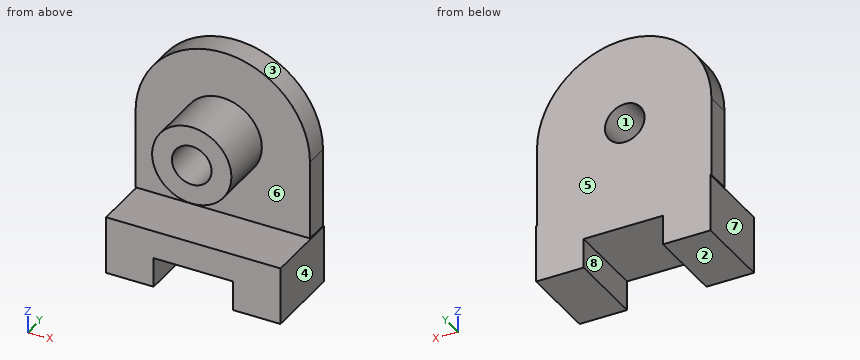
from build123d import *

# Parameters (mm, degrees)
F1_DEPTH = 12
F2_R     = 20
F3_DEPTH = 28
F5_DEPTH = 40
F6_R     = 10
F7_DEPTH = 70


with BuildPart() as f1:
    # F0 (on Front) → F1 (new body)
    with BuildSketch(Plane.XZ):
        with BuildLine():
            Line((44, 0), (44, 40))
            ThreePointArc((44, 40), (0, 84), (-44, 40))
            Line((-44, 40), (-44, 0))
            Line((-44, 0), (44, 0))
        make_face()
    extrude(amount=F1_DEPTH)

    # F2 (on face) → F3 (join)
    with BuildSketch(Plane.XZ.offset(12)):
        with Locations((-0.289364, 40.312858)):
            Circle(F2_R)
    extrude(amount=F3_DEPTH)

    # F4 (on Front) → F5 (join)
    with BuildSketch(Plane.XZ):
        Polygon((44.469752, -29.099998), (44.469752, 0), (-43.530248, 0), (-43.530248, -29.099998), (-19.530248, -29.099998), (-19.530248, -14.099998), (20.469752, -14.099998), (20.469752, -29.099998), align=None)
    extrude(amount=F5_DEPTH)

    # F6 (on face) → F7 (cut)
    with BuildSketch(Plane.XZ.offset(40)):
        with Locations((-0.289364, 40.312858)):
            Circle(F6_R)
    extrude(amount=-F7_DEPTH, mode=Mode.SUBTRACT)


solid = f1.part
The model under review builds one solid part; all positions refer to its coordinate system, in mm. Face numbers are marked on the shaded views. A direction names the side the tool comes from. Coordinates: 2 decimals unless noted, no trailing zeros. Loops run counter-clockwise (first coordinate to the right, second up) from the corner with the lowest first, then second, coordinate; pieces in that order, holes last. Notation, with made-up numbers: M -34.5,30.25 L -26.5,30.25 A24 cw -26.5,45.25 Z; hole C 6.25,-34.5 d1. An arc over 180 degrees is marked long. Put each result on its own line as item: value. Start each with the question number.
Q1. Add section D-D (x = -15). Write out the cut boundary in (y, z), and give its area (3 significant figures).
Q2. The part is to be moulded in two halves that separate along X. For the marked faces 1, 2, 3 and 4, say which applies: +X half, -X half, draft (parallel to the pull), parting line (faces both ways), or undercut.
Q3. Wall thickness on line 1 (Z direction, x = -1, y = -30); line 2 (Z direction, x = -35.5, y = -30.5); line 3 (X direction, y = -10, z = -12): over which ranges is each line inside the solid? List them lowest first.
Q4. Add section B-B (y = -20). Write out the cut boundary in (x, z).
Q5. Add section A-A (z = -17.5). Write out the cut boundary in (x, y).
Q6. Clearance check with flat-ended pins moving along their axes: pin 1 (16.5 mm diameter, centred on y = -18, z = -20, fed in from -X); pin 2 (4 mm diameter, centred on y = -19, z = 26.5, fed in from +X); pin 3 (5 mm diameter, centred on x = 17.5, z = 47.5, fed in from +Y); pin 4 (6 mm diameter, centred on x = -6, y = -26, fed in from -Z). State where each tip first meets the part, or that it passes through.
Q7. Add section C-C (x = 0). Write out the cut boundary in (y, z), and give its area (3 significant figures).
Q8. For the marked faces 5, 6, 7 and 8, list the 3-axis set-ups (+Z, -Z, +X, -X, +Y, -Y) from which the entire face can be reached by the end or side of a thin tool; tool diameter is ignored.
Answers:
1. outline: M -40,-14.1 L 0,-14.1 L 0,81.36 L -12,81.36 L -12,53.86 L -40,53.86 L -40,26.76 L -12,26.76 L -12,0 L -40,0 Z
1. area: 2,300 mm^2
2. face 1: undercut
2. face 2: draft
2. face 3: parting line
2. face 4: +X half
3. line 1: z = -14.1 to 0, 20.33 to 30.34, 50.29 to 60.3
3. line 2: z = -29.1 to 0
3. line 3: x = -43.53 to 44.47
4. outline: M -43.53,-29.1 L -19.53,-29.1 L -19.53,-14.1 L 20.47,-14.1 L 20.47,-29.1 L 44.47,-29.1 L 44.47,0 L -43.53,0 Z; C -0.29,40.31 d40; hole C -0.29,40.31 d20
5. outline: M -43.53,-40 L -19.53,-40 L -19.53,0 L -43.53,0 Z; M 20.47,-40 L 44.47,-40 L 44.47,0 L 20.47,0 Z
6. pin 1: stops at x = -43.53
6. pin 2: stops at x = 15.85
6. pin 3: stops at y = 0
6. pin 4: stops at z = -14.1
7. outline: M -40,-14.1 L 0,-14.1 L 0,30.32 L -40,30.32 L -40,20.31 L -12,20.31 L -12,0 L -40,0 Z; M -40,50.31 L 0,50.31 L 0,84 L -12,84 L -12,60.31 L -40,60.31 Z
7. area: 1,890 mm^2
8. face 5: +Z, -Z, +X, -X, +Y
8. face 6: -Y
8. face 7: -Z, -X, +Y, -Y
8. face 8: -Z, +Y, -Y
